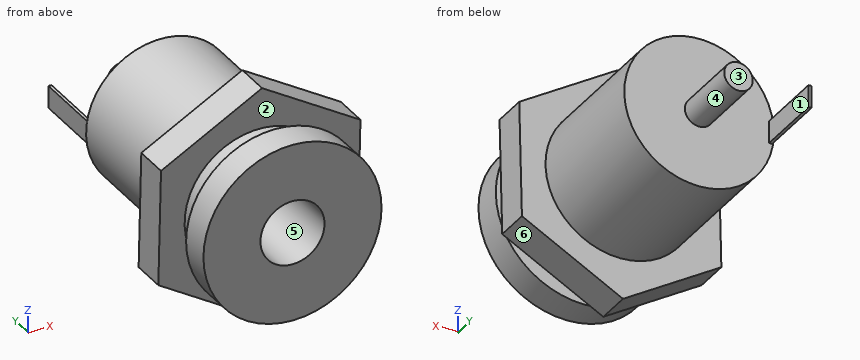
from build123d import *

# Parameters (mm, degrees)
SKETCH_1_R          = 5.25
EXTRUDE_1_DEPTH     = 14.5
SKETCH_2_R          = 1
SKETCH_2_W          = 0.21481542
SKETCH_2_H          = 1.562293966
EXTRUDE_2_DEPTH     = 5
SKETCH_3_R          = 6.25
EXTRUDE_3_DEPTH     = 2.2
EXTRUDE_START       = 2
EXTRUDE_4_DEPTH     = 2.5
SKETCH_5_R          = 2.25
CUT_EXTRUDE_1_DEPTH = 11


with BuildPart() as part:
    # Эскиз1 → Бобышка-Вытянуть1 (new body)
    with BuildSketch(Plane(origin=(0, 0, 0), x_dir=(1, 0, 0), z_dir=(0, 1, 0))):
        with Locations(Location((0, 0, 0), (0, 0, 90))):
            Circle(SKETCH_1_R)
    extrude(amount=EXTRUDE_1_DEPTH)

    # Эскиз2 → Бобышка-Вытянуть2 (add)
    with BuildSketch(Plane(origin=(0, 14.5, 0), x_dir=(1, 0, 0), z_dir=(0, 1, 0))):
        with Locations(Location((0, 0, 0), (0, 0, 270))):
            Circle(SKETCH_2_R)
        with Locations((-5.018869364, 0)):
            Rectangle(SKETCH_2_W, SKETCH_2_H)
    extrude(amount=EXTRUDE_2_DEPTH)

    # Эскиз3 → Бобышка-Вытянуть3 (add)
    with BuildSketch(Plane.XZ):
        with Locations(Location((0, 0, 0), (0, 0, 270))):
            Circle(SKETCH_3_R)
    extrude(amount=EXTRUDE_3_DEPTH)

    # Эскиз4 → Бобышка-Вытянуть4 (add)
    with BuildSketch(Plane(origin=(0, 0, 0), x_dir=(1, 0, 0), z_dir=(0, 1, 0)).offset(EXTRUDE_START)):
        Polygon((7.092328416, -3.877139534), (6.903865539, 4.203566813), (-0.188462877, 8.080706348), (-7.092328416, 3.877139534), (-6.903865539, -4.203566813), (0.188462877, -8.080706348), align=None)
    extrude(amount=EXTRUDE_4_DEPTH)

    # Эскиз5 → Вырез-Вытянуть1 (cut)
    with BuildSketch(Plane.XZ.offset(2.2)):
        with Locations(Location((0, 0, 0), (0, 0, 270))):
            Circle(SKETCH_5_R)
    extrude(amount=-CUT_EXTRUDE_1_DEPTH, mode=Mode.SUBTRACT)


solid = part.part
The listing builds one solid part. Answer for the finished solid, in the listing's coordinates (mm). Face numbers are marked on the shaded views. A direction names the side the tool comes from. Coordinates: 2 decimals unless noted, no trailing zeros. Loops run counter-clockwise (first coordinate to the right, second up) from the corner with the lowest first, then second, coordinate; pieces in that order, holes last. Notation, with made-up numbers: (72, 50.25) -> (129, 50.25) arc R23 cw to (129, 58.25) -> close; hole circle Ø7 at (44, 39). An arc over 180 degrees is marked (long way). Answer in a Markdown table with one row per item. Add a question column.
1. For the marked faces 4, 5 and 6, determine the directions among +Z, -Z, +X, -X, +Y, -Y from which every point of the face is accessible in a straight line to the end or side of a thin tool.
2. Consider line 1 (X direction, y = 5, z = 0); line 2 (Y direction, x = -4, z = -4); line 3 (Y direction, x = 0.25, z = 0.5). Determine where each line is inside the solid, lowest interval first. Write a range as [from, to].
3. The part is cut by section D-D, the plane x = -1.25. Write down the section's boundary in (y, z), then the cut area to 3 significant figures.
4. Determine the mould class of the marked faces 1, 2 and 3 for opening direction Y: +Y half, -Y half, draft (parallel to the pull), parting line (faces both ways), or undercut.
5. The part is cut by section A-A, the plane y = 3.5. Write down the section's boundary in (x, z), then the cut area to 3 significant figures.
6. The part is cut by section B-B, the plane y = 16.5. Write down the section's boundary in (x, z), then the cut area to 3 significant figures.
7. The part is cut by section C-C, the plane z = -1.75. Write down the section's boundary in (x, y), then the cut area to 3 significant figures.
8. Flat-ended cylindrical pins translate along their axes: P1, Ø4.5, axis at x = -1.5, z = -1.5, coming from the +Y side; P2, Ø5, axis at x = -2.5, z = -4, coming from the +Y side; P3, Ø4, axis at x = -3, y = 1, coming from the -Z side; P4, Ø4, axis at x = -1, y = 10, coming from the -Z side. Find the tip coordinate at first contact, or state that the pin passes through.
Answer below:
| question | item | result |
|---|---|---|
| 1 | face 4 | +Y |
| 1 | face 5 | -Y |
| 1 | face 6 | -Z, +X, +Y, -Y |
| 2 | line 1 | [-5.25, -2.25], [2.25, 5.25] |
| 2 | line 2 | [-2.2, 0], [2, 4.5] |
| 2 | line 3 | [8.8, 19.5] |
| 3 | outline | (-2.2, -6.12) -> (0, -6.12) -> (0, -5.1) -> (2, -5.1) -> (2, -7.43) -> (4.5, -7.43) -> (4.5, -5.1) -> (14.5, -5.1) -> (14.5, 5.1) -> (4.5, 5.1) -> (4.5, 7.29) -> (2, 7.29) -> (2, 5.1) -> (0, 5.1) -> (0, 6.12) -> (-2.2, 6.12) -> (-2.2, 1.87) -> (8.8, 1.87) -> (8.8, -1.87) -> (-2.2, -1.87) -> close |
| 3 | area | 145 mm2 |
| 4 | face 1 | draft |
| 4 | face 2 | undercut |
| 4 | face 3 | +Y half |
| 5 | outline | (-7.09, -3.88) -> (-0.19, -8.08) -> (6.9, -4.2) -> (7.09, 3.88) -> (0.19, 8.08) -> (-6.9, 4.2) -> close; hole circle Ø4.5 at (0, 0) |
| 5 | area | 154 mm2 |
| 6 | outline | (-5.13, -0.78) -> (-4.91, -0.78) -> (-4.91, 0.78) -> (-5.13, 0.78) -> close; circle Ø2 at (0, 0) |
| 6 | area | 3.48 mm2 |
| 7 | outline | (-7.04, 2) -> (-4.95, 2) -> (-4.95, 0) -> (-6, 0) -> (-6, -2.2) -> (-1.41, -2.2) -> (-1.41, 8.8) -> (1.41, 8.8) -> (1.41, -2.2) -> (6, -2.2) -> (6, 0) -> (4.95, 0) -> (4.95, 2) -> (6.96, 2) -> (6.96, 4.5) -> (4.95, 4.5) -> (4.95, 14.5) -> (-4.95, 14.5) -> (-4.95, 4.5) -> (-7.04, 4.5) -> close |
| 7 | area | 149 mm2 |
| 8 | P1 | y = 19.5 |
| 8 | P2 | y = 14.5 |
| 8 | P3 | z = -7.42 |
| 8 | P4 | z = -5.25 |
